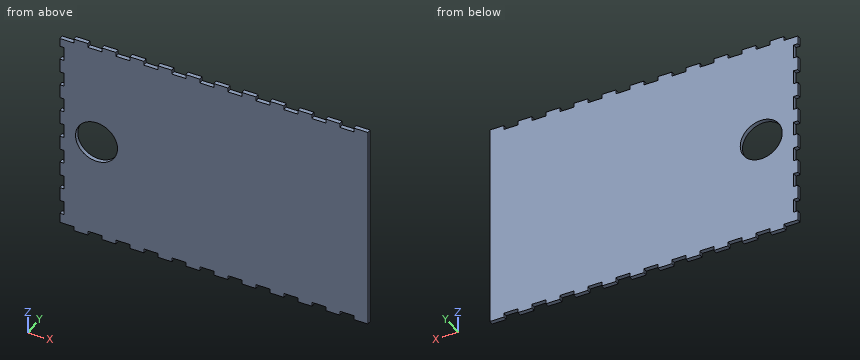
Autodesk Inventor part; units mm, degrees
ref_plane "YZ Plane" through (0, 0, 0) normal (1, 0, 0) x (0, 1, 0)
ref_plane "XZ Plane" through (0, 0, 0) normal (0, 1, 0) x (-1, 0, 0)
ref_plane "XY Plane" through (0, 0, 0) normal (0, 0, 1) x (1, 0, 0)
sketch "Эскиз5" plane through (0, 0, 0) normal (0, 1, 0) x (-1, 0, 0)
  line L0 (-110, 74.5) -> (110, 74.5)
  line L1 (110, 74.5) -> (110, -74.5)
  line L2 (110, -74.5) -> (-110, -74.5)
  line L3 (-110, -74.5) -> (-110, 74.5)
  line L4 (-110, 74.5) -> (110, -74.5) construction
  line L5 (110, 74.5) -> (-110, -74.5) construction
  point P0 (0, 0)
  dimension "d25" = 220
  dimension "d26" = 149
extrude "Выдавливание5" add sketch "Эскиз5" along normal blind 3
sketch "Эскиз6" plane through (0, 3, 0) normal (0, 1, 0) x (1, 0, 0)
  line L0 (-110, 74.5) -> (-110, -74.5)
  line L1 (-110, -65.5) -> (-107, -65.5)
  line L2 (-107, -65.5) -> (-107, -55.5)
  line L3 (-107, -55.5) -> (-110, -55.5)
  line L4 (-110, -55.5) -> (-110, -65.5)
  line L5 (-110, -74.5) -> (110, -74.5)
  point P0 (0, 0)
  point P1 (-107, -74.5)
  point P2 (-110, -65.5)
  dimension "d29" = 3
  dimension "d30" = 10
  dimension "d46" = 9
extrude "Выдавливание6" cut sketch "Эскиз6" against normal blind 3
pattern_linear "Прямоуг.массив6" count 7 spacing 20 along (0, 0, -1) of "Выдавливание6"
sketch "Эскиз8" plane through (0, 3, 0) normal (0, 1, 0) x (1, 0, 0)
  line L0 (-110, -74.5) -> (110, -74.5)
  line L1 (-110, -74.5) -> (-100, -74.5)
  line L2 (-100, -74.5) -> (-100, -71.5)
  line L3 (-100, -71.5) -> (-110, -71.5)
  line L4 (-110, -71.5) -> (-110, -74.5)
  line L5 (-107, -55.5) -> (-107, -65.5)
  point P0 (0, 0)
  dimension "d50" = 3
  dimension "d51" = 10
  dimension "d52" = 3
extrude "Выдавливание8" cut sketch "Эскиз8" against normal blind 3
pattern_linear "Прямоуг.массив7" count 11 spacing 20 along (1, 0, 0) of "Выдавливание8"
mirror "Зеркальное отражение2" about plane through (0, 0, 0) normal (0, 0, 1) of "Выдавливание8", "Прямоуг.массив7"
sketch "Эскиз9" plane through (0, 3, 0) normal (0, 1, 0) x (1, 0, 0)
  circle A0 centre (-83.8133, 0) radius 15
  point P0 (0, 0)
  dimension "d58" = 30
extrude "Выдавливание9" cut sketch "Эскиз9" against normal blind 3
properties part number "000.104 - Cap"
Verification items for the finished model (mm, model axes). Give positions to 0.01 mm unless a question says otherwise; leave off trailing zeros. Write each loop counter-clockwise with the first axis right and the second up, starting at its lowest first coordinate (ties: lowest second). Pieces come first, ordered by that corner, then holes.
(1) Cross-section at A-A (z = 0). Enter the section's corners in (x, y).
(2) Cross-section at B-B (x = 37.5). Enter the section's corners in (y, z).
(3) Material ranges on line 1 (X direction, y = 1.95, z = 0); line 2 (X direction, y = 1.6, z = -57); line 3 (Z direction, x = -73, y = 1.75), recorded low to high.
(4) Gauge pin test, flat ends, axial feed: pin 1 (0.9 mm diameter, centred on y = 1, z = 60, fed in from -X); pin 2 (0.9 mm diameter, centred on y = 2, z = 72.5, fed in from -X); pin 3 (1 mm diameter, centred on x = 14, y = 1.5, fed in from +Z). Record the tip position at first contact, or that the pin passes through.
Worked out:
1. outline: (-107, 0) - (-98.81, 0) - (-98.81, 3) - (-107, 3) - close; (-68.81, 0) - (110, 0) - (110, 3) - (-68.81, 3) - close
2. outline: (0, -71.5) - (3, -71.5) - (3, 71.5) - (0, 71.5) - close
3. line 1: x = -107 to -98.81, -68.81 to 110
3. line 2: x = -107 to 110
3. line 3: z = -74.5 to -10.4, 10.4 to 74.5
4. pin 1: stops at x = -107
4. pin 2: stops at x = -100
4. pin 3: stops at z = 71.5
